Autodesk Inventor part; units mm, degrees
ref_plane "YZ Plane" through (0, 0, 0) normal (1, 0, 0) x (0, 1, 0)
ref_plane "XZ Plane" through (0, 0, 0) normal (0, 1, 0) x (-1, 0, 0)
ref_plane "XY Plane" through (0, 0, 0) normal (0, 0, 1) x (1, 0, 0)
sketch "Sketch1" plane through (0, 0, 0) normal (0, 0, 1) x (1, 0, 0)
  circle A0 centre (0, 0) radius 162.5
  circle A1 centre (0, 0) radius 150
  line L0 (0, 0) -> (0, -162.5) construction
  dimension "outer_diameter" = 325
  dimension "inner_diameter" = 300
extrude "Extrusion1" add sketch "Sketch1" along normal blind 10
sketch "Sketch2" plane through (0, 0, 10) normal (0, 0, 1) x (1, 0, 0)
  arc A0 (136.8569, 72.7681) -> (0, 155) centre (0, 0) ccw construction
  arc A1 (139.285, 74.0591) -> (0, 157.75) centre (0, 0) ccw
  arc A2 (134.4288, 71.477) -> (0, 152.25) centre (0, 0) ccw
  arc A3 (134.4288, 71.477) -> (139.285, 74.0591) centre (136.8569, 72.7681) ccw
  arc A4 (0, 157.75) -> (0, 152.25) centre (0, 155) ccw
  line L0 (0, 0) -> (136.8569, 72.7681) construction
  line L1 (0, 0) -> (0, 155) construction
  line L2 (0, 0) -> (0, -28.237) construction
  arc A5 (-27.393, 155.3534) -> (-150.0292, 48.7474) centre (0, 0) ccw
  arc A6 (-26.4379, 149.937) -> (-144.7984, 47.0478) centre (0, 0) ccw
  arc A7 (-26.4379, 149.937) -> (-27.393, 155.3534) centre (-26.9155, 152.6452) ccw
  arc A8 (-150.0292, 48.7474) -> (-144.7984, 47.0478) centre (-147.4138, 47.8976) ccw
  arc A9 (-156.2148, 21.9546) -> (-92.7231, -127.6224) centre (0, 0) ccw
  arc A10 (-150.7683, 21.1891) -> (-89.4903, -123.1728) centre (0, 0) ccw
  arc A11 (-150.7683, 21.1891) -> (-156.2148, 21.9546) centre (-153.4916, 21.5718) ccw
  arc A12 (-92.7231, -127.6224) -> (-89.4903, -123.1728) centre (-91.1067, -125.3976) ccw
  arc A13 (-69.153, -141.7848) -> (92.7231, -127.6224) centre (0, 0) ccw
  arc A14 (-66.742, -136.8414) -> (89.4903, -123.1728) centre (0, 0) ccw
  arc A15 (-66.742, -136.8414) -> (-69.153, -141.7848) centre (-67.9475, -139.3131) ccw
  arc A16 (92.7231, -127.6224) -> (89.4903, -123.1728) centre (91.1067, -125.3976) ccw
  arc A17 (113.4759, -109.5824) -> (150.0292, 48.7474) centre (0, 0) ccw
  arc A18 (109.5195, -105.7617) -> (144.7984, 47.0478) centre (0, 0) ccw
  arc A19 (109.5195, -105.7617) -> (113.4759, -109.5824) centre (111.4977, -107.672) ccw
  arc A20 (150.0292, 48.7474) -> (144.7984, 47.0478) centre (147.4138, 47.8976) ccw
  point P0 (162.5, 0)
  dimension "slot_radius" = 155
  dimension "slot_length_deg" = 62
  dimension "slot_width" = 5.5
  dimension "d15" = 360
extrude "Extrusion3" cut sketch "Sketch2" against normal blind 10
sketch "Sketch3" plane through (0, 0, 10) normal (0, 0, 1) x (1, 0, 0)
  circle A0 centre (0, 0) radius 150
  circle A1 centre (0, 0) radius 155 construction
  line L0 (0, 0) -> (-13.5091, 154.4102) construction
  arc A2 (0, 157.75) -> (0, 152.25) centre (0, 155) ccw
  line L1 (0, 155) -> (0, 0) construction
  point P0 (-151.0274, 34.8674)
  point P1 (-79.8309, -132.8609)
  point P2 (101.6891, -116.98)
  point P3 (142.6783, 60.5633)
  dimension "d22" = 310
  dimension "d42" = 360
  dimension "d52" = 5
hole "Hole1" at (-13.5091, 154.4102, 10) at (-151.0274, 34.8674, 10) at (-79.8309, -132.8609, 10) at (101.6891, -116.98, 10) at (142.6783, 60.5633, 10) direction (0, 0, -1) diameter 4.134 end through all
sketch "Sketch5" plane through (0, 0, 0) normal (0, 0, -1) x (-1, 0, 0)
  circle A0 centre (0, 0) radius 162.5
  circle A1 centre (0, 0) radius 160
  dimension "d53" = 320
extrude "Extrusion4" cut sketch "Sketch5" against normal blind 8
equation "\"d17\" = thickness"
equation "\"offset_angle_gear\" = 65deg"
properties part number "ytterring"
The listing builds one solid part. Answer for the finished solid, in the listing's coordinates (mm). A direction names the side the tool comes from. Round coordinates to 2 decimals unless told otherwise and drop trailing zeros. Order: outer loops, then holes, each group sorted by start corner. A loop starts at its lowest first (then second) coordinate and runs counter-clockwise, first axis right, second up. Notation, with made-up numbers: (-28, -4.5) -> (15, -4.5) arc R30 ccw to (15, 22.5) -> close; hole circle Ø8 at (-21, 66). An arc over 180 degrees is marked (long way). Put each result on its own line as item: value.
Q1. Determine the mould class of faces 4 (the cylindrical face through (34.685, -156.195, 3.944)), 5 (the cylindrical face through (-102.589, 119.836, 5.07)), 6 (the flat face through (-143, 48, 0)), 7 (the cylindrical face through (12.56, -157.25, 5.07)) for opening direction Y: pulls with the +Y half, pulls with the -Y half, needs draft (parallel to the pull), parting line crosses it, or undercut.
Results list:
face 4: parting line crosses it
face 5: undercut
face 6: needs draft
face 7: undercut
Q2. Each of these flat-tipped pins is pushed along its axis until it touches: P1, Ø3, axis at x = 127.5, z = 2, coming from the +Y side; P2, Ø5, axis at y = -129.5, z = 8, coming from the +X side; P3, Ø5, axis at y = -62.5, z = 2, coming from the +X side; P4, Ø5.5, axis at x = -151.03, y = 34.87, coming from the -Z side. Where does it stop, or does it pass through?
Results list:
P1: y = 98.61
P2: x = 101.38
P3: x = 148.32
P4: z = 0
Q3. Section B-B, the plane x = 63.5 is taken. Write down the section's boundary in (y, z), and give its area (3 significant figures).
Results list:
outline: (-149.58, 8) -> (-146.86, 8) -> (-146.86, 0) -> (-144.41, 0) -> (-144.41, 10) -> (-149.58, 10) -> close; (-138.38, 0) -> (-135.9, 0) -> (-135.9, 10) -> (-138.38, 10) -> close; (135.9, 0) -> (138.38, 0) -> (138.38, 10) -> (135.9, 10) -> close; (144.41, 0) -> (146.86, 0) -> (146.86, 8) -> (149.58, 8) -> (149.58, 10) -> (144.41, 10) -> close
area: 110 mm^2
Q4. Section C-C, the plane z = 2 is taken. Count the separate pieces of the cut face and the enclosed holes in it, and give its area (3 significant figures).
Results list:
separate pieces: 1
enclosed holes: 11
area: 4,940 mm^2
Q5. Section A-A, the plane y = 0 is taken. Write down the section's boundary in (x, z).
Results list:
outline: (-162.5, 8) -> (-160, 8) -> (-160, 0) -> (-157.75, 0) -> (-157.75, 10) -> (-162.5, 10) -> close; (-152.25, 0) -> (-150, 0) -> (-150, 10) -> (-152.25, 10) -> close; (150, 0) -> (152.25, 0) -> (152.25, 10) -> (150, 10) -> close; (157.75, 0) -> (160, 0) -> (160, 8) -> (162.5, 8) -> (162.5, 10) -> (157.75, 10) -> close
Q6. Which of the six approach directions +Z, -Z, +X, -X, +Y, -Y give full straight-line access (tool end or side, diameter ignored) to faces 1 (the flat face through (-73, -132, 10)), 2 (the cylindrical face through (153.434, -36.649, 5.07)), 3 (the flat face through (-120, -108, 8))?
Results list:
face 1: +Z, +X, -X, +Y, -Y
face 2: +Z, -Z
face 3: -Z
Q7. Consider line 1 along X through (y, z) = (-2, 8.75); line 2 along Y through (x, z) = (0, 5.5); line 3 along X through (y, z) = (-10, 0.75). Determine where each line is inside the solid, lowest interval first.
Results list:
line 1: -162.49 to -157.74, -152.24 to -149.99, 149.99 to 152.24, 157.74 to 162.49
line 2: -160 to -157.75, -152.25 to -150, 150 to 152.25, 157.75 to 160
line 3: -159.69 to -157.43, -151.92 to -149.67, 149.67 to 151.92, 157.43 to 159.69
